Input: dimensioned drawing with shaded views. Units: mm. Origin: part minimum x, y, z. Coordinates: 2 decimals unless noted, no trailing zeros. Loops run counter-clockwise (first coordinate to the right, second up) from the corner with the lowest first, then second, coordinate; pieces in that order, holes last. Notation, with made-up numbers: (43, -31) - (61, -31) arc R24 cw to (61, -3) - close; hole circle Ø6 at (56, 70). An arc over 180 degrees is marked (long way). Put each result on its own line as item: value. Start each with the question number.
1) Contact query for flat-ended pins moving along their axis: pin 1 Ø1 at (x, z) = (3.5, 58) entering from -Y; pin 2 Ø2 at (y, z) = (9, 32) entering from -X; pin 3 Ø3 at (x, z) = (3.5, 37.5) entering from +Y; pin 4 Ø3 at (x, z) = (13, 26.5) entering from -Y. Output: stop coordinate, or through.
2) Material intervals for line 1 along Y through (x, z) = (17, 4); line 2 along Y through (x, z) = (18, 48); line 3 along X through (y, z) = (7.25, 94.5), sorted ascending. Write a range as from..to.
3) Section A-A on z = 18. Output: boundary loops of the cut face in (x, y).
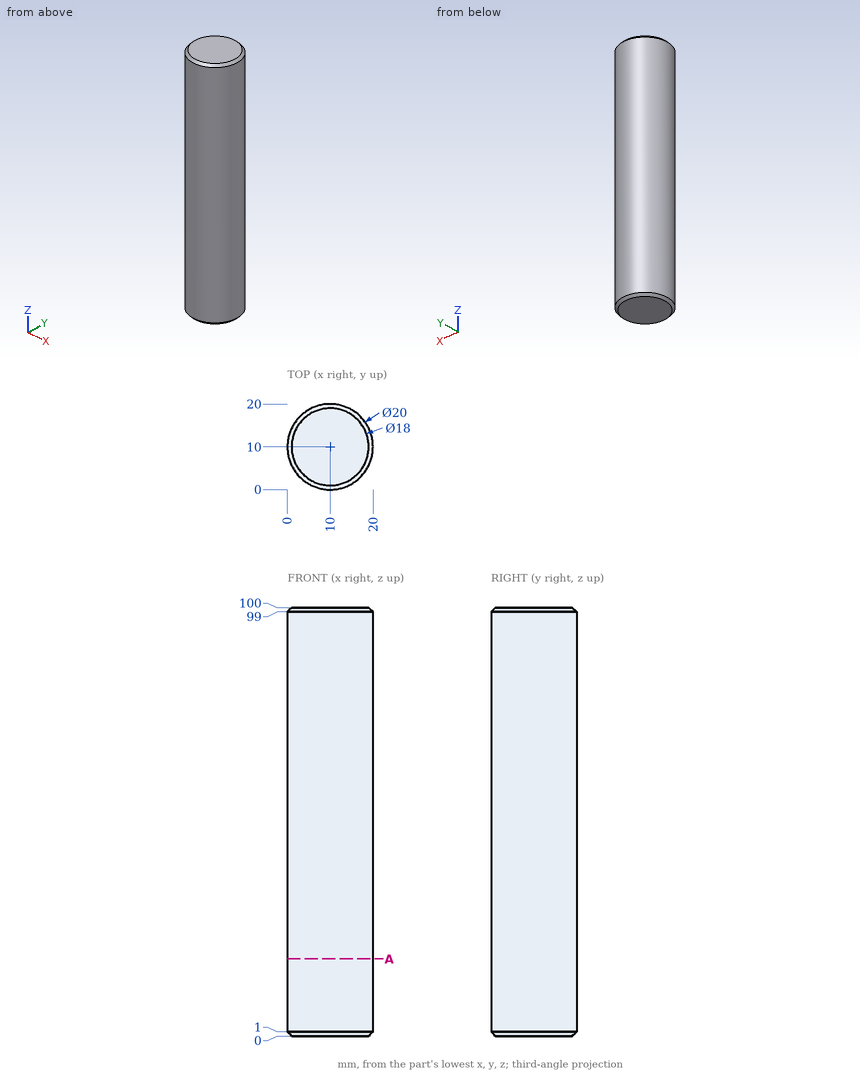
Answer block:
1. pin 1: stops at y = 2
1. pin 2: stops at x = 0
1. pin 3: stops at y = 18.66
1. pin 4: stops at y = 0.11
2. line 1: y = 2.86..17.14
2. line 2: y = 4..16
2. line 3: x = 0.39..19.61
3. outline: circle Ø20 at (10, 10)
